Autodesk Inventor part; units mm, degrees
ref_plane "YZ Plane" through (0, 0, 0) normal (1, 0, 0) x (0, 1, 0)
ref_plane "XZ Plane" through (0, 0, 0) normal (0, 1, 0) x (-1, 0, 0)
ref_plane "XY Plane" through (0, 0, 0) normal (0, 0, 1) x (1, 0, 0)
sketch "スケッチ1" plane through (0, 0, 0) normal (0, 1, 0) x (-1, 0, 0)
  line L0 (-38, 35) -> (38, 35)
  line L1 (38, 35) -> (38, -15)
  line L2 (38, -15) -> (-38, -15)
  line L3 (-38, -15) -> (-38, 35)
  point P0 (0, 0)
  dimension "d0" = 76
  dimension "d3" = 50
  dimension "d4" = 35
  dimension "d5" = 38
extrude "押し出し1" add sketch "スケッチ1" along normal blind 2
sketch "スケッチ2" plane through (0, 2, 0) normal (0, 1, 0) x (1, 0, 0)
  line L0 (-38, -35) -> (38, -35)
  line L1 (38, -35) -> (38, 15)
  line L2 (38, 15) -> (-38, 15)
  line L3 (-38, 15) -> (-38, -35)
  circle A0 centre (-35, 6) radius 1.5
  circle A1 centre (-35, -24) radius 1.5
  circle A2 centre (35, -24) radius 1.5
  circle A3 centre (35, 6) radius 1.5
  point P0 (0, 0)
  dimension "d9" = 3
  dimension "d10" = 30
  dimension "d11" = 70
  dimension "d12" = 70
  dimension "d13" = 3
  dimension "d14" = 11
  dimension "d15" = 30
  dimension "d16" = 3
  dimension "d19" = 11
extrude "押し出し2" cut sketch "スケッチ2" against normal blind 2 keep common part
sketch "スケッチ3" plane through (0, 2, 0) normal (0, 1, 0) x (1, 0, 0)
  circle A0 centre (35, 6) radius 1.5
  line L0 (-38, -35) -> (38, -35)
  line L1 (-38, 15) -> (-38, -35)
  circle A1 centre (-33, 12) radius 1.5
  circle A2 centre (-33, -30) radius 1.5
  circle A3 centre (33, -30) radius 1.5
  circle A4 centre (33, 12) radius 1.5
  point P0 (0, 0)
  dimension "d20" = 66
  dimension "d22" = 42
  dimension "d23" = 42
  dimension "d24" = 66
  dimension "d25" = 5
  dimension "d26" = 5
  dimension "d27" = 5
  dimension "d28" = 5
hole "穴1" at (-33, 2, 30) at (33, 2, 30) at (33, 2, -12) at (-33, 2, -12) direction (0, -1, 0) diameter 3 end through all
properties part number "circuit_plate"
CAD build for the part. Positions are in the model's coordinates, mm. Coordinates: 2 decimals unless noted, no trailing zeros. Order: outer loops, then holes, each group sorted by start corner. A loop starts at its lowest first (then second) coordinate and runs counter-clockwise, first axis right, second up. Notation, with made-up numbers: M 29.5,-6 L 82.5,-6 A21 ccw 82.5,12 Z; hole C 73.5,-25.5 d10. An arc over 180 degrees is marked long. Write each question's results on one line, items separated by ' | '. Start each with the question number.
Q1. Flat gauge pin, fed straight in: P1, Ø2.5, axis at x = -33, z = -12, coming from the +Y side. Where does the tip first touch, or does it go through?
Q2. Drill centre lines: probe 1 along X at (y, z) = (1.1, -6); probe 2 along Z at (x, y) = (-35, 0.8); probe 3 along Z at (x, y) = (-33, 0.65). Where is each one in solid material? Low to high. Write a range as from..to.
Q3. Pull direction X, two halves, no side cores. Call faces 1 (the cylindrical face through (-31.536, 0.986, -12.325)), 2 (the cylindrical face through (33.9, 1, -13.2)), 3 (the flat face through (38, 1, 10)), 4 (the flat face through (1, 1, 35)): +X half, -X half, draft (parallel to the pull), parting line (faces both ways), or undercut.
Q4. Cut at A-A (z = -12). List the corners of the cut face in (x, y), then the cut area to 3 significant figures.
Found:
1) P1: through
2) probe 1: -38..-36.5, -33.5..33.5, 36.5..38 | probe 2: -15..-7.5, -4.5..22.5, 25.5..35 | probe 3: -15..-13.5, -10.5..28.5, 31.5..35
3) face 1: undercut | face 2: undercut | face 3: +X half | face 4: draft
4) outline: M -38,0 L -34.5,0 L -34.5,2 L -38,2 Z; M -31.5,0 L 31.5,0 L 31.5,2 L -31.5,2 Z; M 34.5,0 L 38,0 L 38,2 L 34.5,2 Z | area: 140 mm²
